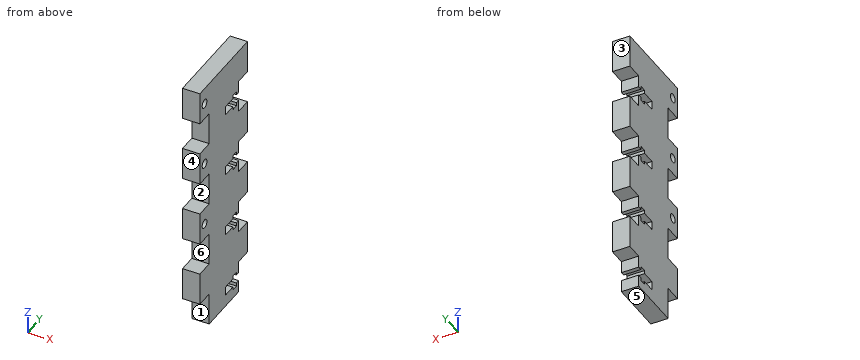
from build123d import *

# Parameters (mm, degrees)
SKETCH1_W           = 96
SKETCH1_H           = 20
BOSS_EXTRUDE1_DEPTH = 6.35
SKETCH2_W           = 12
SKETCH2_H           = 6
SKETCH2_H_2         = 6.35
BOSS_EXTRUDE2_DEPTH = 6.35
SKETCH3_R           = 1.6
CUT_EXTRUDE1_DEPTH  = 10


with BuildPart() as part:
    # Sketch1 → Boss-Extrude1 (new body)
    with BuildSketch(Plane(origin=(0, 0, 0), x_dir=(0, 0, -1), z_dir=(1, 0, 0))):
        Rectangle(SKETCH1_W, SKETCH1_H)
    extrude(amount=BOSS_EXTRUDE1_DEPTH)

    # Sketch2 → Boss-Extrude2 (add)
    with BuildSketch(Plane(origin=(6.35, 0, 0), x_dir=(0, 0, -1), z_dir=(1, 0, 0))):
        with Locations((-18, 13)):
            Rectangle(SKETCH2_W, SKETCH2_H)
        with Locations((-42, 13)):
            Rectangle(SKETCH2_W, SKETCH2_H)
        with Locations((6, 13)):
            Rectangle(SKETCH2_W, SKETCH2_H)
        with Locations((30, 13)):
            Rectangle(SKETCH2_W, SKETCH2_H)
        with Locations((6, -13.175)):
            Rectangle(SKETCH2_W, SKETCH2_H_2)
        with Locations((30, -13.175)):
            Rectangle(SKETCH2_W, SKETCH2_H_2)
        with Locations((-18, -13.175)):
            Rectangle(SKETCH2_W, SKETCH2_H_2)
        with Locations((-42, -13.175)):
            Rectangle(SKETCH2_W, SKETCH2_H_2)
    extrude(amount=-BOSS_EXTRUDE2_DEPTH)

    # Sketch3 → Cut-Extrude1 (cut)
    with BuildSketch(Plane(origin=(6.35, 0, 0), x_dir=(0, 0, -1), z_dir=(1, 0, 0))):
        with Locations((-42, -13.175)):
            Circle(SKETCH3_R)
        with Locations((-18, -13.175)):
            Circle(SKETCH3_R)
        with Locations((6, -13.175)):
            Circle(SKETCH3_R)
        Polygon((-31.6, 10), (-31.6, 8.5), (-32.8, 8.5), (-32.8, 6), (-31.6, 6), (-31.6, 1), (-28.4, 1), (-28.4, 6), (-27.2, 6), (-27.2, 8.5), (-28.4, 8.5), (-28.4, 10), align=None)
        Polygon((-7.6, 10), (-7.6, 8.5), (-8.8, 8.5), (-8.8, 6), (-7.6, 6), (-7.6, 1), (-4.4, 1), (-4.4, 6), (-3.2, 6), (-3.2, 8.5), (-4.4, 8.5), (-4.4, 10), align=None)
        Polygon((16.4, 10), (16.4, 8.5), (15.2, 8.5), (15.2, 6), (16.4, 6), (16.4, 1), (19.6, 1), (19.6, 6), (20.8, 6), (20.8, 8.5), (19.6, 8.5), (19.6, 10), align=None)
        Polygon((40.4, 10), (40.4, 8.5), (39.2, 8.5), (39.2, 6), (40.4, 6), (40.4, 1), (43.6, 1), (43.6, 6), (44.8, 6), (44.8, 8.5), (43.6, 8.5), (43.6, 10), align=None)
    extrude(amount=-CUT_EXTRUDE1_DEPTH, mode=Mode.SUBTRACT)


solid = part.part
The listing builds one solid part. Answer for the finished solid, in the listing's coordinates (mm). Face numbers are marked on the shaded views. A direction names the side the tool comes from. Round coordinates to 2 decimals unless told otherwise and drop trailing zeros. Loops run counter-clockwise (first coordinate to the right, second up) from the corner with the lowest first, then second, coordinate; pieces in that order, holes last. Notation, with made-up numbers: M 14.25,18.25 L 70.25,18.25 A20 ccw 70.25,36.25 Z; hole C 6.25,60.5 d7. An arc over 180 degrees is marked long. Return JSON: item names as keys, results as strings.
Q1. The mould has two halves that part along Z. Classify the marked faces 4, 5 and 6: released by +Z, released by -Z, zero draft, split by the parting line, or undercut.
Results list:
{"face 4": "zero draft", "face 5": "released by -Z", "face 6": "undercut"}
Q2. Which of the six approach directions +Z, -Z, +X, -X, +Y, -Y give full straight-line access (tool end or side, diameter ignored) to the marked faces 1, 2 and 3?
Results list:
{"face 1": "-Z, +X, -X, -Y", "face 2": "+X, -X, -Y", "face 3": "+Z, -Z, +X, -X, +Y"}
Q3. Find section C-C, the plane x = 5.25. State how many separate pieces and enclosed holes the cut face has, plus the area to 3 significant figures.
Results list:
{"separate pieces": "1", "enclosed holes": "3", "area": "2,350 mm2"}
Q4. Each of these flat-tipped pins is pushed along its axis until it touches: pin 1 Ø1.3 at (x, z) = (2, -16) entering from +Y; pin 2 Ø1.3 at (x, z) = (3.5, -20) entering from -Y; pin 3 Ø4 at (y, z) = (-13.175, 18) entering from +X; pin 4 Ø1 at (y, z) = (-12.5, 35) entering from -X. Where does it stop, or does it pass through?
Results list:
{"pin 1": "stops at y = 10", "pin 2": "stops at y = -10", "pin 3": "stops at x = 6.35", "pin 4": "passes through"}
Q5. Find section A-A, the plane z = -6. Determine the outline of the cut face in (x, y) (3 decimals).
Results list:
{"outline": "M 0,-16.35 L 6.35,-16.35 L 6.35,-14.775 L 0,-14.775 Z; M 0,-11.575 L 6.35,-11.575 L 6.35,16 L 0,16 Z"}
Q6. Find section B-B, the plane y = 3. Determine the outline of the cut face in (x, z), plus the area to 3 significant figures.
Results list:
{"outline": "M 0,-48 L 6.35,-48 L 6.35,-43.6 L 0,-43.6 Z; M 0,-40.4 L 6.35,-40.4 L 6.35,-19.6 L 0,-19.6 Z; M 0,-16.4 L 6.35,-16.4 L 6.35,4.4 L 0,4.4 Z; M 0,7.6 L 6.35,7.6 L 6.35,28.4 L 0,28.4 Z; M 0,31.6 L 6.35,31.6 L 6.35,48 L 0,48 Z", "area": "528 mm2"}
Q7. Find the intervals of material crossed by line 1 along Z through (x, y) = (2.5, 2.5); line 2 along Z through (x, y) = (5, 6.5); line 3 along Y through (x, z) = (4, 42) (3 decimals), in increasing order. Write a range as from..to.
Results list:
{"line 1": "z = -48..-43.6, -40.4..-19.6, -16.4..4.4, 7.6..28.4, 31.6..48", "line 2": "z = -48..-44.8, -39.2..-20.8, -15.2..3.2, 8.8..27.2, 32.8..48", "line 3": "y = -16.35..-14.775, -11.575..16"}
